Read the model definition and answer for the solid it produces. Units are mm, in the model's axes. Face numbers are marked on the shaded views. Coordinates: 2 decimals unless noted, no trailing zeros. Order: outer loops, then holes, each group sorted by start corner. A loop starts at its lowest first (then second) coordinate and runs counter-clockwise, first axis right, second up. Notation, with made-up numbers: M 0,-14 L 26,-14 A6 ccw 26,-4 Z; hole C 65.25,-37 d10. An arc over 180 degrees is marked long. One line per question, with ' | ' between items. Start each with the question number.
1) Find section C-C, the plane y = -6.5. Write down the section's boundary in (x, z).
2) The mould has two halves that part along Z. Classify the marked faces 1, 2, 3 and 4: +Z half, -Z half, draft (parallel to the pull), parting line (faces both ways), or undercut.
3) Consider probe 1 along Z at (x, y) = (15.5, -6.6); probe 2 along Z at (x, y) = (0, -7.45); probe 3 along Z at (x, y) = (0, -1.95). Determine where each line is inside the solid, lowest interval first.
4) Given P1, Ø5.5, axis at x = 15.5, z = -15.5, coming from the -Y side; P2, Ø11, axis at x = -3, z = -1, coming from the -Y side, each flat-ended and moving along its own axis, determine where each tip first touches the part or whether it passes through.
5) Find section D-D, the plane z = 0. Write down the section's boundary in (x, y).
6) Find section A-A, the plane x = 15.5. Write down the section's boundary in (y, z).
7) Find section B-B, the plane z = 15.5. Write down the section's boundary in (x, y), plus the area to 3 significant figures.
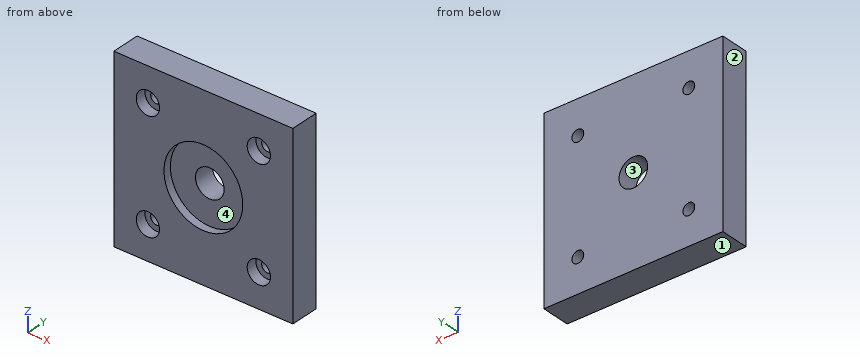
from build123d import *

# Parameters (mm, degrees)
F0_W           = 50
F0_H           = 50
F1_DEPTH       = 8
F3_D           = 8
F3_CBORE_D     = 22
F3_CBORE_DEPTH = 2.2
F5_D           = 3.3
F5_CBORE_D     = 6.5
F5_CBORE_DEPTH = 3


with BuildPart() as f1:
    # F0 (on Front) → F1 (new body)
    with BuildSketch(Plane.XZ):
        Rectangle(F0_W, F0_H)
    extrude(amount=F1_DEPTH)

    # F3 (through all)
    with Locations(Plane.XZ.offset(8)):
        with Locations((0, 0)):
            CounterBoreHole(F3_D / 2, F3_CBORE_D / 2, F3_CBORE_DEPTH)

    # F5 (through all)
    with Locations(Plane.XZ.offset(8)):
        with Locations((15.5, 15.5), (-15.5, 15.5), (-15.5, -15.5), (15.5, -15.5)):
            CounterBoreHole(F5_D / 2, F5_CBORE_D / 2, F5_CBORE_DEPTH)


solid = f1.part
Report:
1) outline: M -25,-25 L 25,-25 L 25,25 L -25,25 Z; hole C -15.5,-15.5 d6.5; hole C -15.5,15.5 d6.5; hole C 0,0 d22; hole C 15.5,-15.5 d6.5; hole C 15.5,15.5 d6.5
2) face 1: -Z half | face 2: draft | face 3: undercut | face 4: undercut
3) probe 1: z = -25 to -18.75, -12.25 to 12.25, 18.75 to 25 | probe 2: z = -25 to -11, 11 to 25 | probe 3: z = -25 to -4, 4 to 25
4) P1: stops at y = -5 | P2: stops at y = -5.8
5) outline: M -25,-8 L -11,-8 L -11,-5.8 L -4,-5.8 L -4,0 L -25,0 Z; M 4,-5.8 L 11,-5.8 L 11,-8 L 25,-8 L 25,0 L 4,0 Z
6) outline: M -8,-25 L 0,-25 L 0,-17.15 L -5,-17.15 L -5,-18.75 L -8,-18.75 Z; M -8,-12.25 L -5,-12.25 L -5,-13.85 L 0,-13.85 L 0,13.85 L -5,13.85 L -5,12.25 L -8,12.25 Z; M -8,18.75 L -5,18.75 L -5,17.15 L 0,17.15 L 0,25 L -8,25 Z
7) outline: M -25,-8 L -18.75,-8 L -18.75,-5 L -17.15,-5 L -17.15,0 L -25,0 Z; M -13.85,-5 L -12.25,-5 L -12.25,-8 L 12.25,-8 L 12.25,-5 L 13.85,-5 L 13.85,0 L -13.85,0 Z; M 17.15,-5 L 18.75,-5 L 18.75,-8 L 25,-8 L 25,0 L 17.15,0 Z | area: 328 mm^2
